Part model, mm, in its own coordinate system. A direction names the side the tool comes from. Round coordinates to 2 decimals unless told otherwise and drop trailing zeros. Write each loop counter-clockwise with the first axis right and the second up, starting at its lowest first coordinate (ties: lowest second). Pieces come first, ordered by that corner, then holes. Notation, with made-up numbers: (13, 84.25) -> (36, 84.25) arc R20 ccw to (36, 123.25) -> close; hole circle Ø6 at (45.25, -22). An arc over 180 degrees is marked (long way). Return JSON: item names as keys, results as strings. Group by question number.
(1) Drop flat-ended pins along their axis: pin 1 Ø1.1 at (y, z) = (46.5, 8) entering from +X; pin 2 Ø1.5 at (x, y) = (43, 54) entering from +Z; pin 3 Ø0.8 at (y, z) = (48, 8) entering from -X. Give the stop position or say it passes through.
(2) Saw through at A-A (x = 106.5). List the corners of the cut face in (y, z).
(3) Drill centre lines: L1, parallel to Z at x = 119, y = 30; L2, parallel to Y at x = 43, z = 6.5; L3, parallel to X at y = 51, z = 6.5. Where is each one in solid material? Low to high. Write a range as from..to.
(4) Saw through at B-B (y = 15.5). List the corners of the cut face in (x, z), plus the area to 3 significant figures.
(5) Tool access for faces 4 (the cylindrical face through (138.99, 2.85, 4.18)), 5 (the cylindrical face through (135.5, 6.5, 7.8)): list every direction of +Z, -Z, +X, -X, +Y, -Y with a clear straight run to the whole face (end or side of a thin tool).
(6) Mould opens along X. For faces 1 (the flat face through (71, 70, 8.3)), 2 (the cylindrical face through (139.15, 69.99, 4.18)), 3 (the cylindrical face through (135.5, 66.5, 7.8)) say: +X half, -X half, draft (parallel to the pull), parting line (faces both ways), or undercut.
Autodesk Inventor part; units mm, degrees
ref_plane "YZ Plane" through (0, 0, 0) normal (1, 0, 0) x (0, 1, 0)
ref_plane "XZ Plane" through (0, 0, 0) normal (0, 1, 0) x (-1, 0, 0)
ref_plane "XY Plane" through (0, 0, 0) normal (0, 0, 1) x (1, 0, 0)
sketch "Sketch1" plane through (0, 0, 0) normal (0, 0, 1) x (1, 0, 0)
  line L0 (0, 0) -> (142, 0)
  line L1 (142, 0) -> (142, 73)
  line L2 (142, 73) -> (0, 73)
  line L3 (0, 73) -> (0, 0)
  dimension "d0" = 142
  dimension "d1" = 73
extrude "Extrusion1" add sketch "Sketch1" along normal blind 8.3
fillet "Fillet1" radius 10 4 edges at (142, 73, 4.15) (142, 0, 4.15) (0, 0, 4.15) (0, 73, 4.15)
fillet "Fillet2" radius 2 16 edges at (2.9289, 70.0711, 8.3) (0, 36.5, 8.3) (2.9289, 2.9289, 8.3) (71, 0, 8.3) (139.0711, 2.9289, 8.3) (142, 36.5, 8.3) (139.0711, 70.0711, 8.3) (71, 73, 8.3) (2.9289, 70.0711, 0) (0, 36.5, 0) (2.9289, 2.9289, 0) (71, 0, 0) (139.0711, 2.9289, 0) (142, 36.5, 0) (139.0711, 70.0711, 0) (71, 73, 0)
sketch "Sketch2" plane through (0, 0, 8.3) normal (0, 0, 1) x (1, 0, 0)
  arc A0 (10, 71) -> (2, 63) centre (10, 63) ccw
  line L0 (2, 10) -> (2, 63)
  arc A1 (2, 10) -> (10, 2) centre (10, 10) ccw
  line L1 (132, 2) -> (10, 2)
  arc A2 (132, 2) -> (140, 10) centre (132, 10) ccw
  line L2 (140, 63) -> (140, 10)
  arc A3 (140, 63) -> (132, 71) centre (132, 63) ccw
  line L3 (10, 71) -> (132, 71)
  arc A4 (136.9512, 63) -> (132, 67.9512) centre (132, 63) ccw
  line L4 (136.9512, 63) -> (136.9512, 10)
  arc A5 (132, 5.0488) -> (136.9512, 10) centre (132, 10) ccw
  line L5 (132, 5.0488) -> (10, 5.0488)
  arc A6 (5.0488, 10) -> (10, 5.0488) centre (10, 10) ccw
  line L6 (5.0488, 10) -> (5.0488, 63)
  arc A7 (10, 67.9512) -> (5.0488, 63) centre (10, 63) ccw
  line L7 (10, 67.9512) -> (132, 67.9512)
  point P0 (0, 0)
extrude "Extrusion2" cut sketch "Sketch2" against normal blind 1 contours L4 A5 L5 A6 L6 A7 L7 A4
properties part number "Phone"
Computed values:
{
 "1": {"pin 1": "x = 141.64", "pin 2": "z = 7.3", "pin 3": "x = 0.48"},
 "2": {"outline": "(0, 2) arc R2 ccw to (2, 0) -> (71, 0) arc R2 ccw to (73, 2) -> (73, 6.3) arc R2 ccw to (71, 8.3) -> (67.95, 8.3) -> (67.95, 7.3) -> (5.05, 7.3) -> (5.05, 8.3) -> (2, 8.3) arc R2 ccw to (0, 6.3) -> close"},
 "3": {"L1": "0..7.3", "L2": "0.01..72.99", "L3": "0.01..141.99"},
 "4": {"outline": "(0, 2) arc R2 ccw to (2, 0) -> (140, 0) arc R2 ccw to (142, 2) -> (142, 6.3) arc R2 ccw to (140, 8.3) -> (136.95, 8.3) -> (136.95, 7.3) -> (5.05, 7.3) -> (5.05, 8.3) -> (2, 8.3) arc R2 ccw to (0, 6.3) -> close", "area": "1,040 mm2"},
 "5": {"face 4": "+Z, -Z, +X, -Y", "face 5": "+Z"},
 "6": {"face 1": "draft", "face 2": "+X half", "face 3": "undercut"}
}
